Part print with two shaded views. Sizes in mm from the minimum x, y, z corner. A direction names the side the tool comes from. Round coordinates to 2 decimals unless told otherwise and drop trailing zeros. Write each loop counter-clockwise with the first axis right and the second up, starting at its lowest first coordinate (ties: lowest second). Pieces come first, ordered by that corner, then holes. Notation, with made-up numbers: (-37, 42.25) - (3, 42.25) arc R24 cw to (3, 54.25) - close; hole circle Ø9 at (41.25, 21.5). An arc over 180 degrees is marked (long way). Use one line per item in the form item = value. Start each with the question number.
Item 1: Pin check, flat tips, straight feed: pin 1 (3 mm diameter, centred on x = 56, z = 4.5, fed in from +Y) (3 decimals); pin 2 (2 mm diameter, centred on y = 6.5, z = 11, fed in from -X); pin 3 (2.5 mm diameter, centred on y = 7.5, z = 9, fed in from +X). Stop position of each tip, or through.
Item 2: Pull direction X, two halves, no side cores. Call the marked faces 4, 5 and 6: +X half, -X half, draft (parallel to the pull), parting line (faces both ways), or undercut.
Item 3: Band-saw the part on B-B, the plane y = 2. Give the number of separate pieces and of enclosed holes in the cut face, and give its area (3 significant figures).
Item 4: Drill centre lines: L1, parallel to Z at x = 58.65, y = 1.65; L2, parallel to X at y = 4, z = 7; L3, parallel to Z at x = 34.29, y = 4.25. Where is each one in solid material? Low to high.
Item 5: Band-saw the part on C-C, the plane x = 57. List the corners of the cut face in (y, z) (1 decimal).
Item 6: Tool access for the marked faces 1, 2 and 3: list every direction of +Z, -Z, +X, -X, +Y, -Y with a clear straight run to the whole face (end or side of a thin tool).
Item 7: Band-saw the part on A-A, the plane z = 6.35. List the corners of the cut face in (x, y) (1 decimal).
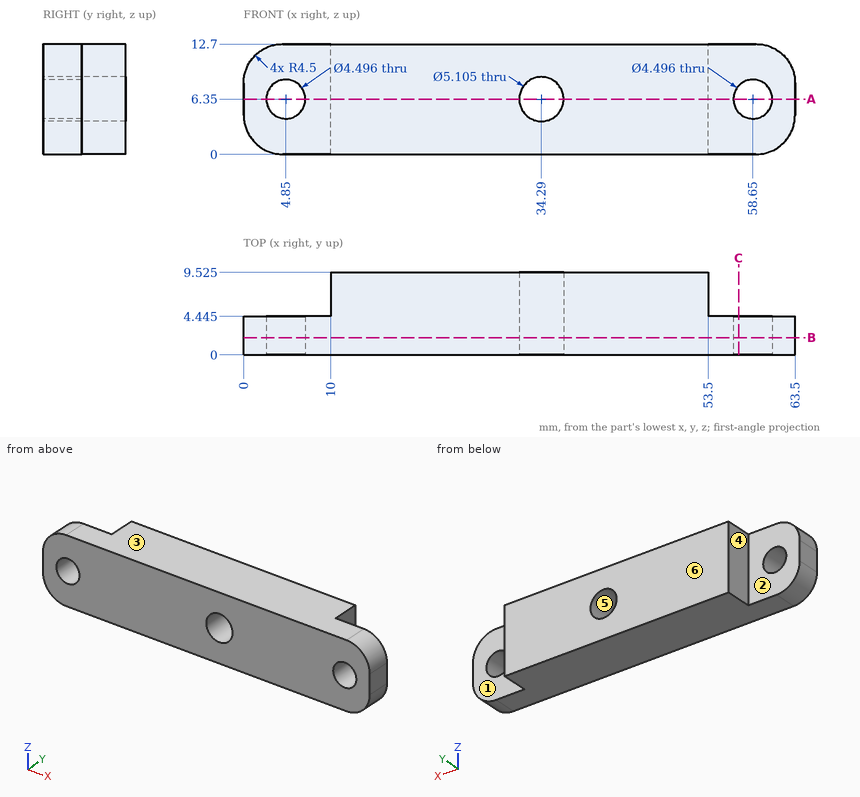
Determined:
q1.pin_1 = 4.445
q1.pin_2 = 10
q1.pin_3 = 53.5
q2.face_4 = -X half
q2.face_5 = undercut
q2.face_6 = draft
q3.separate_pieces = 1
q3.enclosed_holes = 3
q3.area = 737 mm²
q4.L1 = 0 to 4.1, 8.6 to 12.7
q4.L2 = 0 to 2.7, 7 to 31.82, 36.76 to 56.5, 60.8 to 63.5
q4.L3 = 0 to 3.8, 8.9 to 12.7
q5.outline = (0, 0) - (4.4, 0) - (4.4, 4.8) - (0, 4.8) - close; (0, 7.9) - (4.4, 7.9) - (4.4, 12.7) - (0, 12.7) - close
q6.face_1 = +Z, -Z, +X, +Y
q6.face_2 = +Z, -Z, -X, +Y
q6.face_3 = +Z, +X, -X, +Y, -Y
q7.outline = (0, 0) - (2.6, 0) - (2.6, 4.4) - (0, 4.4) - close; (7.1, 0) - (31.7, 0) - (31.7, 9.5) - (10, 9.5) - (10, 4.4) - (7.1, 4.4) - close; (36.8, 0) - (56.4, 0) - (56.4, 4.4) - (53.5, 4.4) - (53.5, 9.5) - (36.8, 9.5) - close; (60.9, 0) - (63.5, 0) - (63.5, 4.4) - (60.9, 4.4) - close
